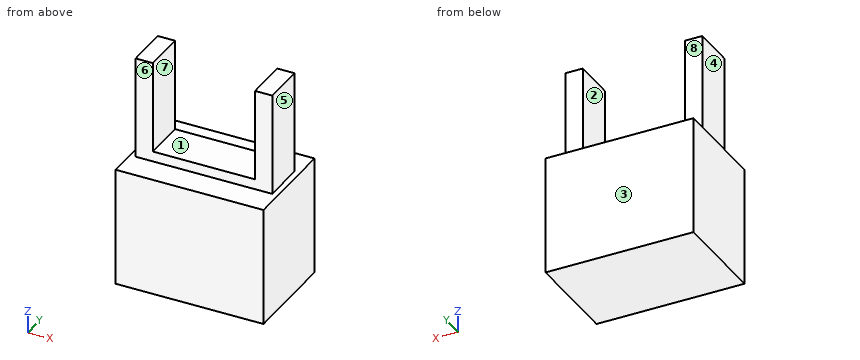
from build123d import *

# Parameters (mm, degrees)
SKETCH1_W           = 101.6
SKETCH1_H           = 31.75
BOSS_EXTRUDE1_DEPTH = 76.2
SKETCH2_W           = 76.064070538
SKETCH2_H           = 31.75
CUT_EXTRUDE1_DEPTH  = 68.58
SKETCH4_W           = 110.036041042
SKETCH4_H           = 73.081165812
BOSS_EXTRUDE2_DEPTH = 88.392


with BuildPart() as part:
    # Sketch1 → Boss-Extrude1 (new body)
    with BuildSketch(Plane.XY):
        Rectangle(SKETCH1_W, SKETCH1_H)
    extrude(amount=BOSS_EXTRUDE1_DEPTH)

    # Sketch2 → Cut-Extrude1 (cut)
    with BuildSketch(Plane.XY.offset(76.2)):
        Rectangle(SKETCH2_W, SKETCH2_H)
    extrude(amount=-CUT_EXTRUDE1_DEPTH, mode=Mode.SUBTRACT)

    # Sketch4 → Boss-Extrude2 (add)
    with BuildSketch(Plane(origin=(0, 0, 0), x_dir=(-1, 0, 0), z_dir=(0, 0, -1))):
        Rectangle(SKETCH4_W, SKETCH4_H)
    extrude(amount=BOSS_EXTRUDE2_DEPTH)


solid = part.part
Work out the finished part from the listing and answer in its coordinate system (mm). Face numbers are marked on the shaded views. A direction names the side the tool comes from. Round coordinates to 2 decimals unless told otherwise and drop trailing zeros. Order: outer loops, then holes, each group sorted by start corner. A loop starts at its lowest first (then second) coordinate and runs counter-clockwise, first axis right, second up. Notation, with made-up numbers: M 49,23.5 L 100,23.5 A14 ccw 100,38.5 Z; hole C 87.25,7 d4. An arc over 180 degrees is marked long. Put each result on its own line as item: value. Start each with the question number.
Q1. For a pull along X with two mould halves and no side action, classify the marked faces 1, 2, 3 and 4 as pulls with the +X half, pulls with the -X half, needs draft (parallel to the pull), parting line crosses it, or undercut.
Q2. Section D-D, the plane x = -6.5 is taken. Write down the section's boundary in (y, z) (3 decimals).
Q3. Section B-B, the plane x = -43.5 is taken. Write down the section's boundary in (y, z) (3 decimals), and give its area (3 significant figures).
Q4. Section C-C, the plane y = 8.5 is taken. Write down the section's boundary in (x, z).
Q5. Straight lines are drawn through the part: L1, parallel to X at y = 2, z = 16; L2, parallel to Z at x = -15, y = 20.5; L3, parallel to Y at x = -14, z = 7 (3 decimals). For each, find the intervals that lie inside material, in ascending order. Write a range as [from, to].
Q6. Flat-ended cylindrical pins translate along their axes: pin 1 (3 mm diameter, centred on x = -21, y = -26, fed in from +Z); pin 2 (2 mm diameter, centred on x = -8.5, y = 1, fed in from +Z); pin 3 (10 mm diameter, centred on x = 31, z = 7.5, fed in from +Y) (3 decimals). Find the tip coordinate at first contact, or state that the pin passes through.
Q7. Section A-A, the plane z = 45.5 is taken. Write down the section's boundary in (x, y) (3 decimals), and give its area (3 significant figures).
Q8. A tool of negligible diameter and unlimited length cuts with its end or side. For the marked faces 5, 6, 7 and 8, from which of +Z, -Z, +X, -X, +Y, -Y can it reach the whole face along a straight path? Write none if from no direction.
Findings below:
1. face 1: undercut
1. face 2: undercut
1. face 3: needs draft
1. face 4: pulls with the -X half
2. outline: M -36.541,-88.392 L 36.541,-88.392 L 36.541,0 L 15.875,0 L 15.875,7.62 L -15.875,7.62 L -15.875,0 L -36.541,0 Z
3. outline: M -36.541,-88.392 L 36.541,-88.392 L 36.541,0 L 15.875,0 L 15.875,76.2 L -15.875,76.2 L -15.875,0 L -36.541,0 Z
3. area: 8,880 mm^2
4. outline: M -55.02,-88.39 L 55.02,-88.39 L 55.02,0 L 50.8,0 L 50.8,76.2 L 38.03,76.2 L 38.03,7.62 L -38.03,7.62 L -38.03,76.2 L -50.8,76.2 L -50.8,0 L -55.02,0 Z
5. L1: x = [-50.8, -38.03], [38.03, 50.8]
5. L2: z = [-88.39, 0]
5. L3: y = [-15.875, 15.875]
6. pin 1: stops at z = 0
6. pin 2: stops at z = 7.62
6. pin 3: stops at y = 15.875
7. outline: M -50.8,-15.875 L -38.032,-15.875 L -38.032,15.875 L -50.8,15.875 Z; M 38.032,-15.875 L 50.8,-15.875 L 50.8,15.875 L 38.032,15.875 Z
7. area: 811 mm^2
8. face 5: +Z, +X, +Y, -Y
8. face 6: +Z, +X, -X, -Y
8. face 7: +Z, +Y, -Y
8. face 8: +Z, +X, -X, +Y
